from build123d import *

# Parameters (mm, degrees)
SKIZZE2_W                       = 240
SKIZZE2_H                       = 120
SKIZZE2_W_2                     = 10
SKIZZE2_H_2                     = 20
SKIZZE2_W_3                     = 20
SKIZZE2_H_3                     = 5
AUFSATZ_LINEAR_AUSTRAGEN1_DEPTH = 5


with BuildPart() as part:
    # Skizze2 → Aufsatz-Linear austragen1 (new body)
    with BuildSketch(Plane(origin=(0, 0, 0), x_dir=(0, 0, -1), z_dir=(1, 0, 0))):
        Rectangle(SKIZZE2_W, SKIZZE2_H)
        with Locations((-125, 50)):
            Rectangle(SKIZZE2_W_2, SKIZZE2_H_2)
        with Locations((125, 50)):
            Rectangle(SKIZZE2_W_2, SKIZZE2_H_2)
        with Locations((-90, -62.5)):
            Rectangle(SKIZZE2_W_3, SKIZZE2_H_3)
        with Locations((90, -62.5)):
            Rectangle(SKIZZE2_W_3, SKIZZE2_H_3)
    extrude(amount=AUFSATZ_LINEAR_AUSTRAGEN1_DEPTH)


solid = part.part
Read the model definition and answer for the solid it produces. Units are mm, in the model's axes. A direction names the side the tool comes from. Coordinates: 2 decimals unless noted, no trailing zeros. Order: outer loops, then holes, each group sorted by start corner. A loop starts at its lowest first (then second) coordinate and runs counter-clockwise, first axis right, second up. Notation, with made-up numbers: M 25,-19.5 L 77,-19.5 A9 cw 77,-15.5 Z; hole C -15.5,74.5 d11. An arc over 180 degrees is marked long. Put each result on its own line as item: value. Start each with the question number.
Item 1: Consider probe 1 along Y at (x, z) = (1, 30.5); probe 2 along Z at (x, y) = (0.7, 19.5). Determine where each line is inside the solid, lowest interval first. Write a range as [from, to].
Item 2: The mould has two halves that part along Z. Classify faces 4 (the face through (2, 40, 125)), 5 (the face through (2, -11, -120)), 6 (the face through (2, -63, -80)), 7 (the face through (2, -63, 80)): +Z half, -Z half, draft (parallel to the pull), parting line (faces both ways), or undercut.
Item 3: Given pin 1 Ø2 at (x, z) = (2.5, 24) entering from -Y; pin 2 Ø1.5 at (x, z) = (3.5, 127) entering from -Y; pin 3 Ø3 at (x, y) = (2.5, -24.5) entering from +Z, each flat-ended and moving along its own axis, determine where each tip first touches the part or whether it passes through.
Item 4: Section A-A, the plane x = 1.15 is taken. Determine the outline of the cut face in (y, z).
Item 5: For faces 1 (the face through (2, -63, 100)), 2 (the face through (2, -60, 1)), 3 (the face through (2, -63, -100)), determine the directions among +Z, -Z, +X, -X, +Y, -Y from which every point of the face is accessible in a straight line to the end or side of a thin tool.
Item 6: Section B-B, the plane z = 5 is taken. Determine the outline of the cut face in (x, y).
Item 7: Section C-C, the plane y = 6 is taken. Determine the outline of the cut face in (x, z), plus the area to 3 significant figures.
Computed:
1. probe 1: y = [-60, 60]
1. probe 2: z = [-120, 120]
2. face 4: draft
2. face 5: -Z half
2. face 6: undercut
2. face 7: undercut
3. pin 1: stops at y = -60
3. pin 2: stops at y = 40
3. pin 3: stops at z = 120
4. outline: M -65,-100 L -60,-100 L -60,-120 L 40,-120 L 40,-130 L 60,-130 L 60,130 L 40,130 L 40,120 L -60,120 L -60,100 L -65,100 L -65,80 L -60,80 L -60,-80 L -65,-80 Z
5. face 1: +Z, +X, -X, -Y
5. face 2: +X, -X, -Y
5. face 3: -Z, +X, -X, -Y
6. outline: M 0,-60 L 5,-60 L 5,60 L 0,60 Z
7. outline: M 0,-120 L 5,-120 L 5,120 L 0,120 Z
7. area: 1,200 mm2
